Source: CAD feature listing. Evaluate the final solid. Frame: model axes, mm. A direction names the side the tool comes from. Coordinates: 2 decimals unless noted, no trailing zeros. Loops run counter-clockwise (first coordinate to the right, second up) from the corner with the lowest first, then second, coordinate; pieces in that order, holes last. Notation, with made-up numbers: (63.25, 12.25) -> (69.25, 12.25) arc R37 ccw to (69.25, 48.25) -> close; hole circle Ø2 at (-17.75, 36.25). An arc over 180 degrees is marked (long way). Answer as CSV lines item,"result".
from build123d import *

# Parameters (mm, degrees)
SKETCH1_W           = 41
SKETCH1_H           = 70
BOSS_EXTRUDE1_DEPTH = 8
FILLET1_R           = 4
CHAMFER1_SIZE       = 1
SKETCH2_R           = 3.3
CUT_EXTRUDE1_DEPTH  = 8
CHAMFER2_SIZE       = 3.2
SKETCH3_R           = 5.5
CUT_EXTRUDE2_DEPTH  = 4.2
SKETCH4_R           = 5.1
CUT_EXTRUDE3_DEPTH  = 10
SKETCH5_R           = 10
CUT_EXTRUDE5_DEPTH  = 4
SKETCH6_R           = 10
BOSS_EXTRUDE2_DEPTH = 8


with BuildPart() as part:
    # Sketch1 → Boss-Extrude1 (new body)
    with BuildSketch(Plane(origin=(0, 0, 0), x_dir=(1, 0, 0), z_dir=(0, 1, 0))):
        Rectangle(SKETCH1_W, SKETCH1_H)
    extrude(amount=BOSS_EXTRUDE1_DEPTH)

    # Fillet1
    fillet1_edges = [part.edges().sort_by_distance(p)[0] for p in [
        (20.5, 4, 35),
        (-20.5, 4, 35),
        (-20.5, 4, -35),
        (20.5, 4, -35),
    ]]
    fillet(fillet1_edges, radius=FILLET1_R)

    # Chamfer1
    chamfer1_edges = [part.edges().sort_by_distance(p)[0] for p in [
        (-20.5, 0, 0),
        (-20.5, 8, 0),
        (20.5, 0, 0),
        (0, 0, 35),
        (0, 0, -35),
        (-19.328427125, 0, 33.828427125),
        (19.328427125, 0, 33.828427125),
        (19.328427125, 0, -33.828427125),
        (-19.328427125, 0, -33.828427125),
        (0, 8, -35),
        (20.5, 8, 0),
        (0, 8, 35),
        (-19.328427125, 8, 33.828427125),
        (19.328427125, 8, 33.828427125),
        (19.328427125, 8, -33.828427125),
        (-19.328427125, 8, -33.828427125),
    ]]
    chamfer(chamfer1_edges, length=CHAMFER1_SIZE)

    # Sketch2 → Cut-Extrude1 (cut)
    with BuildSketch(Plane(origin=(0, 8, 0), x_dir=(1, 0, 0), z_dir=(0, 1, 0))):
        with Locations((0, -17.5)):
            Circle(SKETCH2_R)
        with Locations((0, 17.5)):
            Circle(SKETCH2_R)
    extrude(amount=-CUT_EXTRUDE1_DEPTH, mode=Mode.SUBTRACT)

    # Chamfer2
    chamfer2_edges = [part.edges().sort_by_distance(p)[0] for p in [
        (-3.3, 8, 17.5),
    ]]
    chamfer(chamfer2_edges, length=CHAMFER2_SIZE)

    # Sketch3 → Cut-Extrude2 (cut)
    with BuildSketch(Plane(origin=(0, 8, 0), x_dir=(1, 0, 0), z_dir=(0, 1, 0))):
        with Locations((0, 17.5)):
            Circle(SKETCH3_R)
    extrude(amount=-CUT_EXTRUDE2_DEPTH, mode=Mode.SUBTRACT)

    # Sketch4 → Cut-Extrude3 (cut)
    with BuildSketch(Plane(origin=(0, 8, 0), x_dir=(1, 0, 0), z_dir=(0, 1, 0))):
        Circle(SKETCH4_R)
    extrude(amount=-CUT_EXTRUDE3_DEPTH, mode=Mode.SUBTRACT)

    # Sketch5 → Cut-Extrude5 (cut)
    with BuildSketch(Plane(origin=(0, 8, 0), x_dir=(1, 0, 0), z_dir=(0, 1, 0))):
        Circle(SKETCH5_R)
    extrude(amount=-CUT_EXTRUDE5_DEPTH, mode=Mode.SUBTRACT)

    # Sketch6 → Boss-Extrude2 (add)
    with BuildSketch(Plane(origin=(0, 8, 0), x_dir=(1, 0, 0), z_dir=(0, 1, 0))):
        Circle(SKETCH6_R)
    extrude(amount=-BOSS_EXTRUDE2_DEPTH)


solid = part.part
(1) Cut plane C-C (y = 2.25). Return the cut outline in (x, z), then the cut area to 3 significant figures.
Computed values:
outline,"(-20.5, -31) arc R4 ccw to (-16.5, -35) -> (16.5, -35) arc R4 ccw to (20.5, -31) -> (20.5, 31) arc R4 ccw to (16.5, 35) -> (-16.5, 35) arc R4 ccw to (-20.5, 31) -> close; hole circle Ø6.6 at (0, -17.5); hole circle Ø6.6 at (0, 17.5)"
area,"2,790 mm^2"
(2) Draft query along Z for faces 3 (the cylindrical face through (-0.72, 1.93, -14.28)), 4 (the cylindrical face through (19.359, 4.042, -33.797)), 5 (the cylindrical face through (-19.359, 4.042, 33.797)), 6 (the flat face through (20.5, 4, 0)). Return one class per face: released by +Z, released by -Z, zero draft, split by the parting line, or undercut.
Computed values:
face 3,"undercut"
face 4,"released by -Z"
face 5,"released by +Z"
face 6,"zero draft"
(3) Cut plane B-B (z = 17.5). Return the cut outline in (x, y), then the cut area to 3 significant figures.
Computed values:
outline,"(-20.5, 1) -> (-19.5, 0) -> (-3.3, 0) -> (-3.3, 4.8) -> (-6.5, 8) -> (-19.5, 8) -> (-20.5, 7) -> close; (3.3, 0) -> (19.5, 0) -> (20.5, 1) -> (20.5, 7) -> (19.5, 8) -> (6.5, 8) -> (3.3, 4.8) -> close"
area,"263 mm^2"
(4) Cut plane A-A (x = 0). Return the cut outline in (y, z), then the cut area to 3 significant figures.
Computed values:
outline,"(0, -34) -> (1, -35) -> (7, -35) -> (8, -34) -> (8, -23) -> (3.8, -23) -> (3.8, -20.8) -> (0, -20.8) -> close; (0, -14.2) -> (3.8, -14.2) -> (3.8, -12) -> (8, -12) -> (8, 11) -> (4.8, 14.2) -> (0, 14.2) -> close; (0, 20.8) -> (4.8, 20.8) -> (8, 24) -> (8, 34) -> (7, 35) -> (1, 35) -> (0, 34) -> close"
area,"424 mm^2"
(5) Cut plane D-D (z = -17.5). Return the cut outline in (x, y).
Computed values:
outline,"(-20.5, 1) -> (-19.5, 0) -> (-3.3, 0) -> (-3.3, 3.8) -> (-5.5, 3.8) -> (-5.5, 8) -> (-19.5, 8) -> (-20.5, 7) -> close; (3.3, 0) -> (19.5, 0) -> (20.5, 1) -> (20.5, 7) -> (19.5, 8) -> (5.5, 8) -> (5.5, 3.8) -> (3.3, 3.8) -> close"
(6) Pin query (flat end, axial travel): pin 1 Ø8.5 at (x, z) = (0, 17.5) entering from +Y; pin 2 Ø5.5 at (x, z) = (-1, -18.5) entering from +Y. Return the tip coordinate at first contact, or that it passes through.
Computed values:
pin 1,"y = 5.75"
pin 2,"y = 3.8"
(7) Access query for faces 1 (the cylindrical face through (-4.05, 5.93, -21.22)), 2 (the flat face through (0, 0, 0)). Directions: +Z, -Z, +X, -X, +Y, -Y. A direction counts if a zero-diameter tool reaches every point of the face in a straight line with its end or side. Return the directions, or none.
Computed values:
face 1,"+Y"
face 2,"+Z, -Z, +X, -X, -Y"
(8) Material intervals for L1, parallel to Z at x = 0, y = 1.6; L2, parallel to X at y = 3.2, z = 17.5; L3, parallel to Z at x = 0, y = 5.6, sorted ascending. Write a range as [from, to].
Computed values:
L1,"[-35, -20.8], [-14.2, 14.2], [20.8, 35]"
L2,"[-20.5, -3.3], [3.3, 20.5]"
L3,"[-35, -23], [-12, 13.4], [21.6, 35]"
